```python
from build123d import *

# Parameters (mm, degrees)
F0_W     = 116.989415
F0_H     = 48.217313
F1_DEPTH = 25.4
F3_DEPTH = 116.990415
F4_R     = 0.254


with BuildPart() as f1:
    # F0 (on Top) → F1 (new body)
    with BuildSketch(Plane.XY):
        with Locations((2.449287, 1.776933)):
            Rectangle(F0_W, F0_H)
    extrude(amount=F1_DEPTH)

    # F2 (on face) → F3 (cut, through all)
    with BuildSketch(Plane.YZ.offset(60.943995)):
        Polygon((-15.981724, 5.67151), (-9.631724, 0), (13.185589, 0), (19.535589, 5.67151), align=None)
    extrude(amount=-F3_DEPTH, mode=Mode.SUBTRACT)

    # F4
    f4_edges = [f1.edges().sort_by_distance(p)[0] for p in [
        (2.449287, -15.981724, 5.67151),
        (2.449287, 19.535589, 5.67151),
    ]]
    fillet(f4_edges, radius=F4_R)


solid = f1.part
```
The listing builds one solid part. Answer for the finished solid, in the listing's coordinates (mm). A direction names the side the tool comes from. Coordinates: 2 decimals unless noted, no trailing zeros. Write each loop counter-clockwise with the first axis right and the second up, starting at its lowest first coordinate (ties: lowest second). Pieces come first, ordered by that corner, then holes. Notation, with made-up numbers: (73, -28) - (102, -28) arc R23 cw to (102, -17) - close; hole circle Ø10 at (19.5, -24.5). An arc over 180 degrees is marked (long way). One line per item, written item: value.
1) For a pull along Z with two mould halves and no side action, classify faces 1 (the flat face through (2, 2, 25.4)), 2 (the flat face through (3.268, 16.071, 2.577)), 3 (the flat face through (3.27, -12.6, 2.65)), 4 (the flat face through (-56.045, 1, 15)) as pulls with the +Z half, pulls with the -Z half, needs draft (parallel to the pull), parting line crosses it, or undercut.
Geometry check:
face 1: pulls with the +Z half
face 2: undercut
face 3: undercut
face 4: needs draft
2) This flat-tipped pin is pushed along its axis until it touches: pin 1 Ø1 at (x, y) = (13.5, 10.5) entering from -Z. Where does it stop, or does it pass through?
Geometry check:
pin 1: stops at z = 5.67
3) Find section A-A (x = 37.5). Give the vertices of the cut face in (y, z), and give its area (3 significant figures).
Geometry check:
outline: (-22.33, 0) - (-9.63, 0) - (-15.49, 5.23) arc R0.25 cw to (-15.32, 5.67) - (18.87, 5.67) arc R0.25 cw to (19.04, 5.23) - (13.19, 0) - (25.89, 0) - (25.89, 25.4) - (-22.33, 25.4) - close
area: 1,060 mm2
4) A tool of negligible diameter and unlimited length cuts with its end or side. For faces 5 (the flat face through (3, 2, 5.672)), 6 (the flat face through (2, -22.332, 13)), from which of +Z, -Z, +X, -X, +Y, -Y can it reach the whole face along a straight path? Write none if from no direction.
Geometry check:
face 5: +X, -X
face 6: +Z, -Z, +X, -X, -Y
5) Find section C-C (y = -2). Give the vertices of the cut face in (x, z).
Geometry check:
outline: (-56.05, 5.67) - (60.94, 5.67) - (60.94, 25.4) - (-56.05, 25.4) - close
6) Find section B-B (y = 14.5). Give the vertices of the cut face in (x, z), and give its area (3 significant figures).
Geometry check:
outline: (-56.05, 0) - (60.94, 0) - (60.94, 1.17) - (-56.05, 1.17) - close; (-56.05, 5.67) - (60.94, 5.67) - (60.94, 25.4) - (-56.05, 25.4) - close
area: 2,450 mm2
7) Consider line 1 along Z through (x, y) = (13, 7); line 2 along Y through (x, z) = (-11, 5.5). Determine where each line is inside the solid, lowest interval first. Write a range as from..to.
Geometry check:
line 1: z = 5.67..25.4
line 2: y = -22.33..-15.56, 19.11..25.89
